Here's the drawing with two shaded views (mm, measured from the low corner). I have some questions. Give positions to 0.01 mm unless a question says otherwise; leave off trailing zeros. Order: outer loops, then holes, each group sorted by start corner. A loop starts at its lowest first (then second) coordinate and runs counter-clockwise, first axis right, second up. Notation, with made-up numbers: M -25.75,-18 L -15.75,-18 A26 cw -15.75,-3 Z; hole C 78,-39.5 d1. An arc over 180 degrees is marked long. One line per question, with ' | ' between items. Start each with the question number.
1) If we section it at B-B, the plane y = 37.5: Please give me the cut outline in (x, z), plus the area to 3 significant figures.
2) If we section it at D-D, the plane x = 23: Please give me the cut outline in (y, z).
3) Please list where these lines run through material, in increasing order: line 1 along Y through (x, z) = (5.5, 11.75) (1 decimal); line 2 along X through (y, z) = (46, 9.25); line 3 along X through (y, z) = (51.5, 3.5) (1 decimal). Write a range as [from, to].
4) If we section it at A-A, the plane x = 32: Please give me the cut outline in (y, z), plus the area to 3 significant figures.
5) I'm going to push a flat-ended pin straight in: pin 1 Ø10 at (x, z) = (13, 9.5) entering from +Y. Where does the tip first touch, or does it pass through?
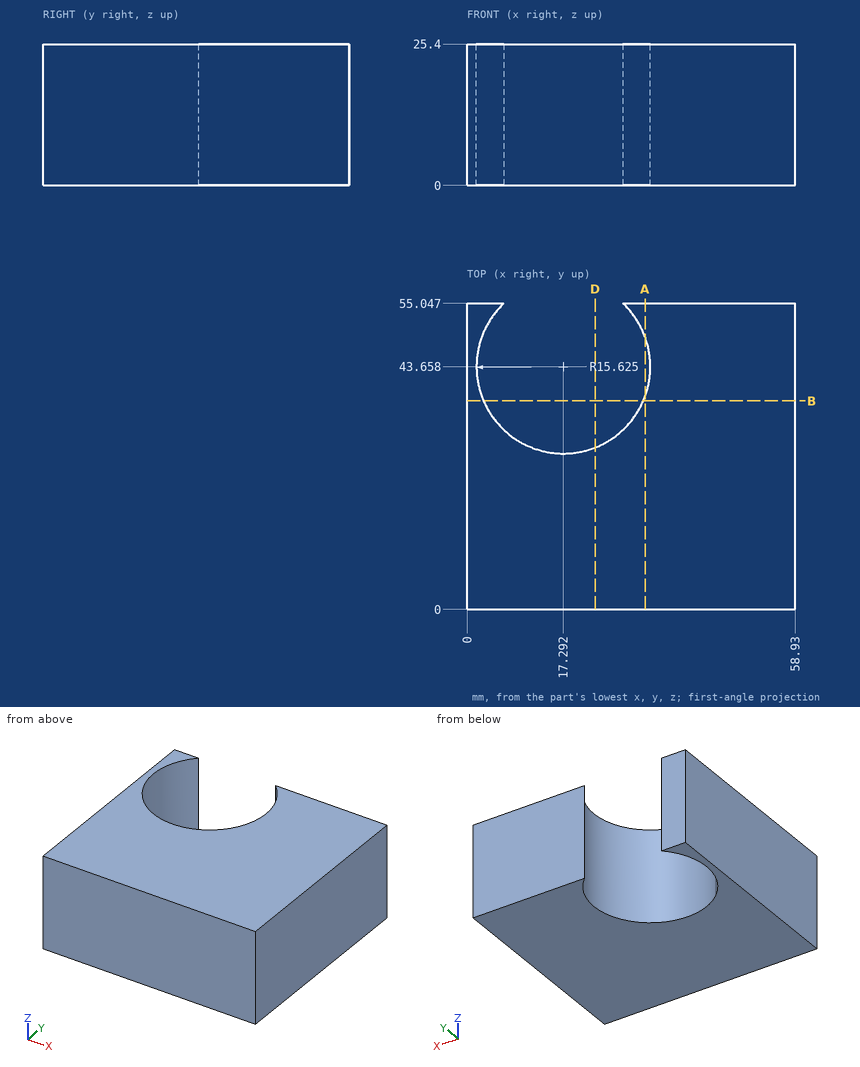
Results found:
1) outline: M 0,0 L 2.93,0 L 2.93,25.4 L 0,25.4 Z; M 31.65,0 L 58.93,0 L 58.93,25.4 L 31.65,25.4 Z | area: 767 mm²
2) outline: M 0,0 L 29.11,0 L 29.11,25.4 L 0,25.4 Z
3) line 1: y = [0, 33.4], [53.9, 55] | line 2: x = [0, 1.84], [32.74, 58.93] | line 3: x = [0, 3.8], [30.8, 58.9]
4) outline: M 0,0 L 38.39,0 L 38.39,25.4 L 0,25.4 Z; M 48.93,0 L 55.05,0 L 55.05,25.4 L 48.93,25.4 Z | area: 1,130 mm²
5) pin 1: stops at y = 31.1
